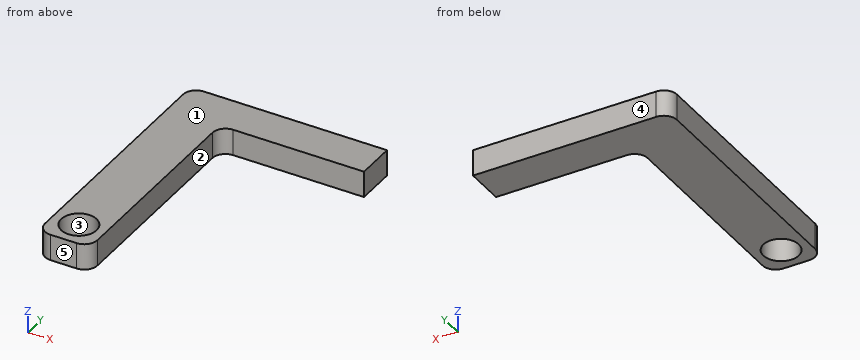
from build123d import *

# Parameters (mm, degrees)
SKETCH1_W           = 40
SKETCH1_H           = 170
BOSS_EXTRUDE1_DEPTH = 20
SKETCH2_W           = 150
SKETCH2_H           = 20
BOSS_EXTRUDE2_DEPTH = 30
FILLET1_R           = 10
CUT_EXTRUDE1_REACH  = 22
SKETCH3_R           = 13.5
FILLET2_R           = 10


with BuildPart() as part:
    # Sketch1 → Boss-Extrude1 (new body)
    with BuildSketch(Plane.XY):
        Rectangle(SKETCH1_W, SKETCH1_H)
    extrude(amount=BOSS_EXTRUDE1_DEPTH)

    # Sketch2 → Boss-Extrude2 (add)
    with BuildSketch(Plane(origin=(0, 85, 0), x_dir=(1, 0, 0), z_dir=(0, 1, 0))):
        with Locations((55, -10)):
            Rectangle(SKETCH2_W, SKETCH2_H)
    extrude(amount=BOSS_EXTRUDE2_DEPTH)

    # Fillet1
    fillet1_edges = [part.edges().sort_by_distance(p)[0] for p in [
        (20, -85, 10),
        (-20, -85, 10),
        (-20, 115, 10),
    ]]
    fillet(fillet1_edges, radius=FILLET1_R)

    # Sketch3 → Cut-Extrude1 (cut, up to next)
    with BuildSketch(Plane.XY.offset(20), mode=Mode.PRIVATE) as cut_extrude1_sk1:
        with Locations((0, -65)):
            Circle(SKETCH3_R)
    cut_extrude1_tool1 = extrude(cut_extrude1_sk1.sketch, amount=-CUT_EXTRUDE1_REACH, mode=Mode.PRIVATE) & part.part
    add(cut_extrude1_tool1.solids().sort_by_distance((0, -65, 20))[0], mode=Mode.SUBTRACT)

    # Fillet2
    fillet2_edges = [part.edges().sort_by_distance(p)[0] for p in [
        (20, 85, 10),
    ]]
    fillet(fillet2_edges, radius=FILLET2_R)


solid = part.part
Design review of the part built by this model. Coordinates are the model's own, in mm. Face numbers are marked on the shaded views. A direction names the side the tool comes from. Give positions to 0.01 mm unless a question says otherwise; leave off trailing zeros. Order: outer loops, then holes, each group sorted by start corner. A loop starts at its lowest first (then second) coordinate and runs counter-clockwise, first axis right, second up. Notation, with made-up numbers: (-11, 66) - (17, 66) arc R9 ccw to (17, 76) - close; hole circle Ø8 at (71, 59). An arc over 180 degrees is marked (long way). Use CSV: the item, a comma, the result in double quotes. Start each with the question number.
Q1. Take a section at A-A (y = -65). State the section outline as (x, z) points.
Q2. Take a section at B-B (z = 2.5). State the section outline as (x, y) points.
Q3. Draft analysis for pull direction Y (two halves, no side actions). For the marked faces 3, 4 and 5, state which applies: pulls with the +Y half, pulls with the -Y half, needs draft (parallel to the pull), parting line crosses it, or undercut.
Q4. For P1, Ø10, axis at x = 103, z = 7, coming from the -Y side; P2, Ø10, axis at y = -33, z = 7, coming from the +X side, all flat-tipped, find the tip position at first contact; note any pin that passes through.
Q5. For line 1 (Y direction, x = 0, z = 9.5); line 2 (X direction, y = 11.5, z = 3.25); line 3 (Y direction, x = 110.5, z = 6.75), list the stretches that pass through material, from the lowest coordinate up.
Q6. Take a section at C-C (x = 0). State the section outline as (y, z) points, and give its area (3 significant figures).
Q7. Take a section at D-D (x = 78.5). State the section outline as (y, z) points.
Q8. Machinability: for the marked faces 1 and 2, which of the approach directions +Z, -Z, +X, -X, +Y, -Y give a long, thin tool a straight path to every point of the face, cutting with its end or side? Answer none if there is none.
Calculated:
1,outline,"(-20, 0) - (-13.5, 0) - (-13.5, 20) - (-20, 20) - close; (13.5, 0) - (20, 0) - (20, 20) - (13.5, 20) - close"
2,outline,"(-20, -75) arc R10 ccw to (-10, -85) - (10, -85) arc R10 ccw to (20, -75) - (20, 75) arc R10 cw to (30, 85) - (130, 85) - (130, 115) - (-10, 115) arc R10 ccw to (-20, 105) - close; hole circle Ø27 at (0, -65)"
3,face 3,"undercut"
3,face 4,"pulls with the +Y half"
3,face 5,"pulls with the -Y half"
4,P1,"stops at y = 85"
4,P2,"stops at x = 20"
5,line 1,"y = -85 to -78.5, -51.5 to 115"
5,line 2,"x = -20 to 20"
5,line 3,"y = 85 to 115"
6,outline,"(-85, 0) - (-78.5, 0) - (-78.5, 20) - (-85, 20) - close; (-51.5, 0) - (115, 0) - (115, 20) - (-51.5, 20) - close"
6,area,"3,460 mm²"
7,outline,"(85, 0) - (115, 0) - (115, 20) - (85, 20) - close"
8,face 1,"+Z, +X, -X, +Y, -Y"
8,face 2,"+Z, -Z, +X, -Y"
